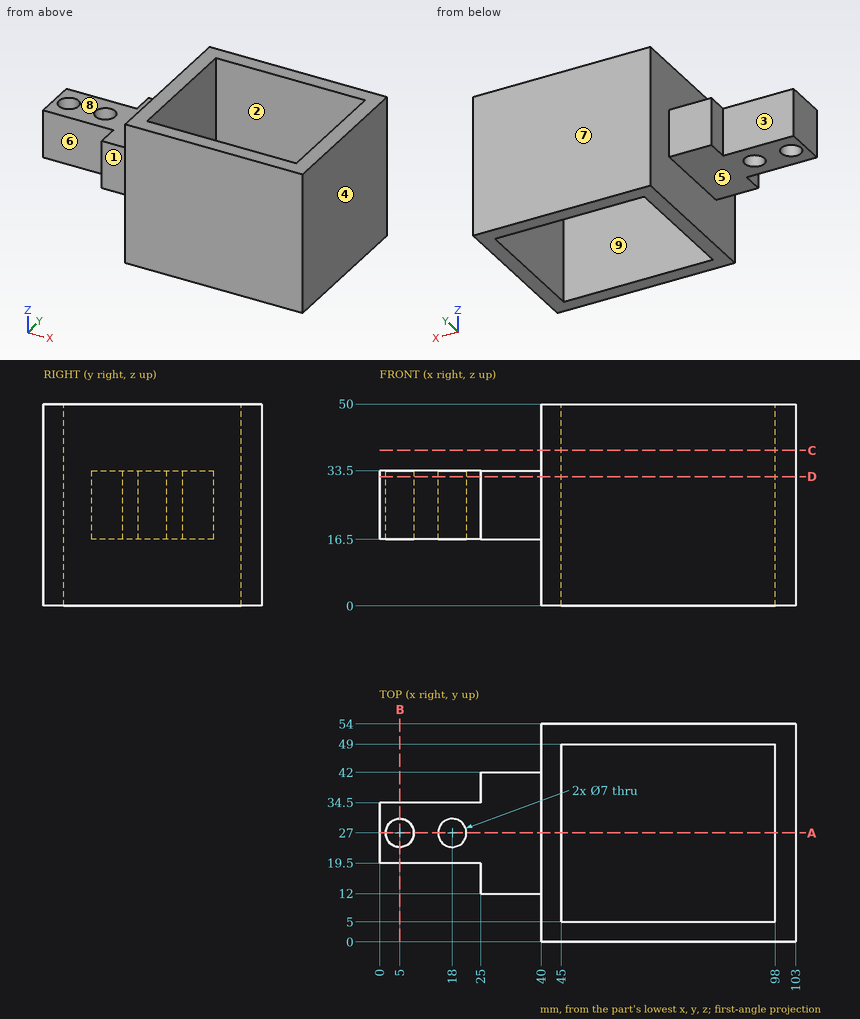
Check sheet for the drawn part. Datum: minimum x, y, z corner. Units: mm. A direction names the side the tool comes from. Coordinates: 2 decimals unless noted, no trailing zeros. Order: outer loops, then holes, each group sorted by start corner. A loop starts at its lowest first (then second) coordinate and runs counter-clockwise, first axis right, second up. Notation, with made-up numbers: (37.25, 57) -> (78.25, 57) arc R22 cw to (78.25, 65) -> close; hole circle Ø4 at (63.25, -17.75). An arc over 180 degrees is marked (long way). Use a Markdown table: item, result. Add a question column.
1. Cross-section at C-C (z = 38.5). Enter the section's corners in (x, y).
2. Mould release check, pull along Y, two halves, no side actions. Record for the marked faces 6, 7, 8 and 9: pulls with the +Y half, pulls with the -Y half, needs draft (parallel to the pull), parting line crosses it, or undercut.
3. Set-up check for the marked faces 1, 2, 3, 4 and 5: record each of +Z, -Z, +X, -X, +Y, -Y from which the full face is reachable in a straight line by a thin tool's end or side.
4. Cross-section at A-A (y = 27). Enter the section's corners in (x, z), and give its area (3 significant figures).
5. Material ranges on L1, parallel to X at y = 35, z = 16; L2, parallel to Y at x = 18, z = 30; L3, parallel to X at y = 25, z = 19, recorded low to high.
6. Cross-section at B-B (x = 5). Enter the section's corners in (y, z).
7. Go/stop test with flat-tipped pins: pin 1 Ø4 at (y, z) = (17, 23) entering from -X; pin 2 Ø15 at (x, z) = (61.5, 29.5) entering from -Y; pin 3 Ø15 at (x, y) = (12, 25) entering from +Z; pin 4 Ø18.5 at (x, z) = (12.5, 25.5) entering from +Y. Record where each tip stops, or that it passes through.
8. Cross-section at D-D (z = 32). Enter the section's corners in (x, y).
Filled sheet:
| question | item | result |
|---|---|---|
| 1 | outline | (40, 0) -> (103, 0) -> (103, 54) -> (40, 54) -> close; hole (45, 5) -> (98, 5) -> (98, 49) -> (45, 49) -> close |
| 2 | face 6 | pulls with the -Y half |
| 2 | face 7 | pulls with the +Y half |
| 2 | face 8 | needs draft |
| 2 | face 9 | undercut |
| 3 | face 1 | +Z, -Z, -X, -Y |
| 3 | face 2 | +Z, -Z |
| 3 | face 3 | +Z, -Z, -X, +Y |
| 3 | face 4 | +Z, -Z, +X, +Y, -Y |
| 3 | face 5 | -Z, -X, +Y, -Y |
| 4 | outline | (0, 16.5) -> (1.5, 16.5) -> (1.5, 33.5) -> (0, 33.5) -> close; (8.5, 16.5) -> (14.5, 16.5) -> (14.5, 33.5) -> (8.5, 33.5) -> close; (21.5, 16.5) -> (40, 16.5) -> (40, 0) -> (45, 0) -> (45, 50) -> (40, 50) -> (40, 33.5) -> (21.5, 33.5) -> close; (98, 0) -> (103, 0) -> (103, 50) -> (98, 50) -> close |
| 4 | area | 942 mm2 |
| 5 | L1 | 40 to 45, 98 to 103 |
| 5 | L2 | 19.5 to 23.5, 30.5 to 34.5 |
| 5 | L3 | 0 to 2.13, 7.87 to 15.13, 20.87 to 45, 98 to 103 |
| 6 | outline | (19.5, 16.5) -> (23.5, 16.5) -> (23.5, 33.5) -> (19.5, 33.5) -> close; (30.5, 16.5) -> (34.5, 16.5) -> (34.5, 33.5) -> (30.5, 33.5) -> close |
| 7 | pin 1 | x = 25 |
| 7 | pin 2 | y = 0 |
| 7 | pin 3 | z = 33.5 |
| 7 | pin 4 | y = 34.5 |
| 8 | outline | (0, 19.5) -> (25, 19.5) -> (25, 12) -> (40, 12) -> (40, 0) -> (103, 0) -> (103, 54) -> (40, 54) -> (40, 42) -> (25, 42) -> (25, 34.5) -> (0, 34.5) -> close; hole circle Ø7 at (5, 27); hole circle Ø7 at (18, 27); hole (45, 5) -> (98, 5) -> (98, 49) -> (45, 49) -> close |
